Can you work these out from the model? Positions are in its coordinate system, mm. A direction names the side the tool comes from. Coordinates: 2 decimals unless noted, no trailing zeros. Order: outer loops, then holes, each group sorted by start corner. A loop starts at its lowest first (then second) coordinate and runs counter-clockwise, first axis right, second up. Notation, with made-up numbers: (89, 81.25) -> (136, 81.25) arc R17 ccw to (136, 102.25) -> close; hole circle Ø11 at (71, -24.75). An arc over 180 degrees is marked (long way). Use a Markdown table: item, result. Add a question column.
1. Suppose I cut it at B-B, the plane x = -4.25. List the corners of the cut face in (y, z) for me.
2. For pin 1 Ø4 at (y, z) = (0, 9) entering from -X; pin 2 Ø0.9 at (y, z) = (1, 0) entering from +X; pin 3 Ø2 at (x, z) = (7.5, 26) entering from -Y, each with a flat end and sliding along its axis, tell me the tip position at first contact or that it passes through.
3. If I drill on line 1 along Y through (x, z) = (0.75, 2); line 2 along Z through (x, y) = (3.75, -0.25); line 3 along Y through (x, z) = (-8.5, 20), over which ranges is the centre line in solid material (lowest first)? Write a range as from..to.
4. For faces 1 (the flat face through (-3.21, -0.32, 0.39)), 2 (the cylindrical face through (10.671, 0.016, 1.157)), 3 (the cylindrical face through (11.106, 3.41, 18.516)), 4 (the cylindrical face through (-11.106, 3.41, 18.516)), which set-ups out of +Z, -Z, +X, -X, +Y, -Y let a thin tool reach every point of the face, with its end or its side?
5. We'd pull the mould along X, two halves only. Please class faces 5 (the cylindrical face through (10.534, 2.85, 18.52)), 6 (the cylindrical face through (11.241, 0.016, 0.595)), 7 (the cylindrical face through (-11.106, -3.41, 18.516)): pulls with the +X half, pulls with the -X half, needs draft (parallel to the pull), parting line crosses it, or undercut.
6. Suppose I cut it at A-A, the plane x = -1.5. List the corners of the cut face in (y, z) for me.
```python
from build123d import *
from OCP.BRepFilletAPI import BRepFilletAPI_MakeFillet

# Parameters (mm, degrees)
SKETCH2_W           = 23.6
SKETCH2_H           = 8.3
BOSS_EXTRUDE1_DEPTH = 34.6
BOSS_EXTRUDE1_DRAFT = -0.5
FILLET1_R1          = 2
FILLET1_R2          = 3
SHELL1_T            = -0.8
CUT_EXTRUDE1_DEPTH  = 33.85


with BuildPart() as part:
    # Sketch2 → Boss-Extrude1 (with draft: the straight prism first)
    with BuildSketch(Plane.XY):
        Rectangle(SKETCH2_W, SKETCH2_H)
    extrude(amount=BOSS_EXTRUDE1_DEPTH)
    # Boss-Extrude1: the draft: its side faces are tilted about the plane it starts from
    boss_extrude1_sides = [part.faces().sort_by_distance(p)[0] for p in [
        (0, -4.15, 17.3),
        (11.8, 0, 17.3),
        (0, 4.15, 17.3),
        (-11.8, 0, 17.3),
    ]]
    draft(boss_extrude1_sides, Plane.XY, BOSS_EXTRUDE1_DRAFT)

    # Fillet1: one fillet with a radius per group of edges: ONE call of the kernel's fillet builder (fillet() takes one radius for all edges)
    fillet1_edges_1 = [part.edges().sort_by_distance(p)[0] for p in [
        (0, -4.15, 0),
        (-11.8, 0, 0),
        (0, 4.15, 0),
        (11.8, 0, 0),
    ]]
    fillet1_edges_2 = [part.edges().sort_by_distance(p)[0] for p in [
        (11.950974813, -4.300974813, 17.3),
        (-11.950974813, -4.300974813, 17.3),
        (-11.950974813, 4.300974813, 17.3),
        (11.950974813, 4.300974813, 17.3),
    ]]
    fillet1 = BRepFilletAPI_MakeFillet(part.part.solid().wrapped)
    for e in fillet1_edges_1:
        fillet1.Add(FILLET1_R1, e.wrapped)
    for e in fillet1_edges_2:
        fillet1.Add(FILLET1_R2, e.wrapped)
    add(Compound.cast(fillet1.Shape()), mode=Mode.REPLACE)

    # Shell1
    shell1_openings = [part.faces().sort_by_distance(p)[0] for p in [
        (0, 0, 34.6),
    ]]
    offset(amount=SHELL1_T, openings=shell1_openings, kind=Kind.INTERSECTION)

    # Sketch3 → Cut-Extrude1 (cut)
    with BuildSketch(Plane(origin=(0, 0, 0), x_dir=(-1, 0, 0), z_dir=(0, 0, -1))):
        with BuildLine():
            Line((3.01539715, 2.217301425), (-3.05, 2.217301425))
            ThreePointArc((-3.05, 2.217301425), (-3.626903312, 1.989192787), (-3.867301425, 1.417301425))
            Line((-3.867301425, 1.417301425), (-3.867301425, 0.541731715))
            ThreePointArc((-3.867301425, 0.541731715), (-3.820065179, 0.308381695), (-3.685793986, 0.111773604))
            Line((-3.685793986, 0.111773604), (-2.807954647, -0.742656685))
            ThreePointArc((-2.807954647, -0.742656685), (-2.615321704, -0.868564956), (-2.389462086, -0.912698575))
            Line((-2.389462086, -0.912698575), (2.354859236, -0.912698575))
            ThreePointArc((2.354859236, -0.912698575), (2.580718854, -0.868564956), (2.773351797, -0.742656685))
            Line((2.773351797, -0.742656685), (3.651191136, 0.111773604))
            ThreePointArc((3.651191136, 0.111773604), (3.776159697, 0.310381805), (3.81539715, 0.541731715))
            Line((3.81539715, 0.541731715), (3.81539715, 1.417301425))
            ThreePointArc((3.81539715, 1.417301425), (3.581082575, 1.98298685), (3.01539715, 2.217301425))
        make_face()
    extrude(amount=-CUT_EXTRUDE1_DEPTH, mode=Mode.SUBTRACT)


solid = part.part
```
Worked out:
| question | item | result |
|---|---|---|
| 1 | outline | (-4.45, 34.6) -> (-4.17, 1.98) arc R2 ccw to (-2.17, 0) -> (2.17, 0) arc R2 ccw to (4.17, 1.98) -> (4.45, 34.6) -> (3.65, 34.6) -> (3.37, 1.99) arc R1.2 cw to (2.17, 0.8) -> (-2.17, 0.8) arc R1.2 cw to (-3.37, 1.99) -> (-3.65, 34.6) -> close |
| 2 | pin 1 | stops at x = -11.9 |
| 2 | pin 2 | stops at x = 11.08 |
| 2 | pin 3 | stops at y = -4.39 |
| 3 | line 1 | y = -4.17..-3.37, 3.37..4.17 |
| 3 | line 2 | z = 0..0.8 |
| 3 | line 3 | y = -4.32..-3.52, 3.52..4.32 |
| 4 | face 1 | +Z, -Z |
| 4 | face 2 | +Z |
| 4 | face 3 | -Z, +X, +Y |
| 4 | face 4 | -Z, -X, +Y |
| 5 | face 5 | undercut |
| 5 | face 6 | pulls with the +X half |
| 5 | face 7 | pulls with the -X half |
| 6 | outline | (-4.45, 34.6) -> (-4.17, 1.98) arc R2 ccw to (-2.17, 0) -> (-0.91, 0) -> (-0.91, 0.8) -> (-2.17, 0.8) arc R1.2 cw to (-3.37, 1.99) -> (-3.65, 34.6) -> close; (2.22, 0) arc R2 ccw to (4.17, 1.98) -> (4.45, 34.6) -> (3.65, 34.6) -> (3.37, 1.99) arc R1.2 cw to (2.22, 0.8) -> close |
